```python
from build123d import *

# Parameters (mm, degrees)
PAD001_DEPTH         = 53.3
PAD002_DEPTH         = 53.3
POCKET_DEPTH         = 19
POCKET001_DEPTH      = 5
POCKET004_DEPTH      = 20.401
POCKET004_DEPTH_BACK = -2.101
FILLET_R             = 2
FILLET001_R          = 1


with BuildPart() as part:
    # Sketch001 → Pad001 (new body, symmetric)
    with BuildSketch(Plane.XZ):
        Polygon((64.25, 0), (55.9, 0), (55.9, -20.4), (-55.3, -20.4), (-55.3, 0), (-64.25, 0), (-64.25, 2.1), (-53.3, 2.1), (-53.3, -17.9), (53.3, -17.9), (53.3, 2.1), (64.25, 2.1), align=None)
    extrude(amount=PAD001_DEPTH, both=True)

    # Sketch002 → Pad002 (join, symmetric)
    with BuildSketch(Plane.XZ):
        with BuildLine():
            ThreePointArc((53, 2.1), (52.25, 1.35), (53, 0.6))
            Line((53.3, 0.6), (53, 0.6))
            Line((53.3, 2.1), (53.3, 0.6))
            Line((53.3, 2.1), (53, 2.1))
        make_face()
    pad002 = extrude(amount=PAD002_DEPTH, both=True)

    # Sketch003 → Pocket (cut)
    with BuildSketch(Plane.XY):
        with BuildLine():
            ThreePointArc((28.8, 39.3), (40.3, 27.8), (51.8, 39.3))
            Line((51.8, 39.3), (51.8, 48.3))
            ThreePointArc((51.8, 48.3), (51.214214, 49.714214), (49.8, 50.3))
            Line((30.8, 50.3), (49.8, 50.3))
            ThreePointArc((30.8, 50.3), (29.385786, 49.714214), (28.8, 48.3))
            Line((28.8, 39.3), (28.8, 48.3))
        make_face()
        with BuildLine():
            ThreePointArc((51.8, -39.3), (40.3, -27.8), (28.8, -39.3))
            Line((28.8, -39.3), (28.8, -48.3))
            ThreePointArc((28.8, -48.3), (29.385786, -49.714214), (30.8, -50.3))
            Line((30.8, -50.3), (49.8, -50.3))
            ThreePointArc((49.8, -50.3), (51.214214, -49.714214), (51.8, -48.3))
            Line((51.8, -39.3), (51.8, -48.3))
        make_face()
    pocket = extrude(amount=-POCKET_DEPTH, mode=Mode.SUBTRACT)

    # Mirrored: Pad002, Pocket across Sketch002 V_Axis
    add(pad002.mirror(Plane(origin=(0, 0, 0), x_dir=(0, -1, 0), z_dir=(1, 0, 0))))
    add(pocket.mirror(Plane(origin=(0, 0, 0), x_dir=(0, -1, 0), z_dir=(1, 0, 0))), mode=Mode.SUBTRACT)

    # Sketch004 → Pocket001 (cut)
    with BuildSketch(Plane.XY):
        with BuildLine():
            ThreePointArc((59.55, -45.8), (59.803187, -46.603007), (60.471172, -47.11557))
            Line((60.471172, -47.11557), (64.25, -48.490951))
            Line((64.25, -42.959049), (64.25, -48.490951))
            Line((60.471172, -44.33443), (64.25, -42.959049))
            ThreePointArc((60.471172, -44.33443), (59.803187, -44.846993), (59.55, -45.65))
            Line((59.55, -45.65), (59.55, -45.8))
        make_face()
        with BuildLine():
            ThreePointArc((60.471172, 47.11557), (59.803187, 46.603007), (59.55, 45.8))
            Line((59.55, 45.8), (59.55, 45.65))
            ThreePointArc((59.55, 45.65), (59.803187, 44.846993), (60.471172, 44.33443))
            Line((60.471172, 44.33443), (64.25, 42.959049))
            Line((64.25, 48.490951), (64.25, 42.959049))
            Line((60.471172, 47.11557), (64.25, 48.490951))
        make_face()
    pocket001 = extrude(amount=POCKET001_DEPTH, mode=Mode.SUBTRACT)

    # Mirrored001: Pocket001 across YZ
    add(pocket001.mirror(Plane.YZ), mode=Mode.SUBTRACT)

    # Sketch005 → Pocket004 (cut, two sides)
    with BuildSketch(Plane.XY) as pocket004_sk:
        Polygon((47.3, -7.5), (47.3, 7.5), (53.3, 7.5), (55.3, 6.5), (55.3, -6.5), (53.3, -7.5), align=None)
    extrude(amount=-POCKET004_DEPTH, mode=Mode.SUBTRACT)
    extrude(pocket004_sk.sketch, amount=-POCKET004_DEPTH_BACK, mode=Mode.SUBTRACT)

    # Fillet
    fillet_edges = [part.edges().sort_by_distance(p)[0] for p in [
        (64.25, -53.3, 1.05),
        (64.25, 53.3, 1.05),
        (-64.25, 53.3, 1.05),
        (-64.25, -53.3, 1.05),
    ]]
    fillet(fillet_edges, radius=FILLET_R)

    # Fillet001
    fillet001_edges = [part.edges().sort_by_distance(p)[0] for p in [
        (55.3, 6.5, -9.15),
        (47.3, 7.5, -19.15),
        (47.3, -7.5, -19.15),
        (55.3, -6.5, -9.15),
    ]]
    fillet(fillet001_edges, radius=FILLET001_R)


solid = part.part
```
Input: part model. Units: mm. Frame: model coordinates. A direction names the side the tool comes from. Round coordinates to 2 decimals unless told otherwise and drop trailing zeros. Loops run counter-clockwise (first coordinate to the right, second up) from the corner with the lowest first, then second, coordinate; pieces in that order, holes last. Notation, with made-up numbers: M -25,41 L 21,41 A8 cw 21,52 Z; hole C 65,31 d1. An arc over 180 degrees is marked long. Answer in a Markdown table with one row per item. Add a question column.
1. Contact query for flat-ended pins moving along their axis: pin 1 (1.2 mm diameter, centred on y = 42.5, z = -18.5, fed in from -X); pin 2 (3 mm diameter, centred on y = 0.5, z = -19.5, fed in from +X); pin 3 (2 mm diameter, centred on x = 21.5, y = -29.5, fed in from +Z). Output: stop coordinate, or through.
2. Section A-A (y = -41). Output: boundary loops of the cut face in (x, z), and give its area (3 significant figures).
3. Section B-B (x = -40.3). Output: boundary loops of the cut face in (y, z).
4. Ray query, probe 1 along X at (y, z) = (36, -2.25); probe 2 along X at (y, z) = (2, -1); probe 3 along Y at (x, z) = (32, -18.5). Return the intervals inside material, ascending.
5. Set-up query: faces 1 (the face through (-60, -1, 0)), 2 (the face through (40.047, 27.803, -18.442)), 3 (the face through (53.3, -31, -9)), 4 (the face through (60, -1, 0)), 5 (the face through (55.3, 0, -9)). Return all of +Z, -Z, +X, -X, +Y, -Y with unobstructed straight access to the full face (end or side cutting, diameter ignored); none if empty.
6. Section C-C (z = -5.5). Output: boundary loops of the cut face in (x, y), and give its area (3 significant figures).
7. Mould query, pull axis Y, two halves, no side actions, for faces 6 (the face through (55.9, -1, -10)), 7 (the face through (0, 53.3, -19)), 8 (the face through (40, 39, -19)). Classes: released by +Y, released by -Y, zero draft, split by the parting line, or undercut.
8. Section D-D (y = 24.5). Output: boundary loops of the cut face in (x, z), and give its area (3 significant figures).
Values follow:
| question | item | result |
|---|---|---|
| 1 | pin 1 | x = -55.3 |
| 1 | pin 2 | x = 55.9 |
| 1 | pin 3 | z = -17.9 |
| 2 | outline | M -64.25,0 L -55.3,0 L -55.3,-20.4 L 55.9,-20.4 L 55.9,0 L 64.25,0 L 64.25,2.1 L 53,2.1 A0.75 ccw 53,0.6 L 53.3,0.6 L 53.3,-17.9 L 51.8,-17.9 L 51.8,-19 L 28.8,-19 L 28.8,-17.9 L -28.8,-17.9 L -28.8,-19 L -51.8,-19 L -51.8,-17.9 L -53.3,-17.9 L -53.3,0.6 L -53,0.6 A0.75 ccw -53,2.1 L -64.25,2.1 Z |
| 2 | area | 358 mm^2 |
| 3 | outline | M -53.3,-20.4 L 53.3,-20.4 L 53.3,-17.9 L 50.3,-17.9 L 50.3,-19 L 27.8,-19 L 27.8,-17.9 L -27.8,-17.9 L -27.8,-19 L -50.3,-19 L -50.3,-17.9 L -53.3,-17.9 Z |
| 4 | probe 1 | -55.3 to -53.3, 53.3 to 55.9 |
| 4 | probe 2 | -55.3 to -53.3, 55.3 to 55.9 |
| 4 | probe 3 | -53.3 to -50.3, -31.34 to 31.34, 50.3 to 53.3 |
| 5 | face 1 | -Z, -X, +Y, -Y |
| 5 | face 2 | +Z |
| 5 | face 3 | +Y, -Y |
| 5 | face 4 | -Z, +X, +Y, -Y |
| 5 | face 5 | +Z, -Z |
| 6 | outline | M -55.3,-53.3 L -53.3,-53.3 L -53.3,53.3 L -55.3,53.3 Z; M 53.3,-53.3 L 55.9,-53.3 L 55.9,53.3 L 53.3,53.3 L 53.3,7.5 L 54.75,6.78 A1 cw 55.3,5.88 L 55.3,-5.88 A1 cw 54.75,-6.78 L 53.3,-7.5 Z |
| 6 | area | 462 mm^2 |
| 7 | face 6 | zero draft |
| 7 | face 7 | released by +Y |
| 7 | face 8 | undercut |
| 8 | outline | M -64.25,0 L -55.3,0 L -55.3,-20.4 L 55.9,-20.4 L 55.9,0 L 64.25,0 L 64.25,2.1 L 53,2.1 A0.75 ccw 53,0.6 L 53.3,0.6 L 53.3,-17.9 L -53.3,-17.9 L -53.3,0.6 L -53,0.6 A0.75 ccw -53,2.1 L -64.25,2.1 Z |
| 8 | area | 409 mm^2 |
